Input: part model. Units: mm. Frame: model coordinates. Face numbers are marked on the shaded views. A direction names the side the tool comes from. Give positions to 0.01 mm unless a question says otherwise; leave off trailing zeros. Order: outer loops, then holes, each group sorted by start corner. A loop starts at its lowest first (then second) coordinate and runs counter-clockwise, first axis right, second up. Notation, with made-up numbers: M 17,-25.75 L 35,-25.75 A19 cw 35,-13.75 Z; hole C -28,62 d11. An arc over 180 degrees is marked long. Use a Markdown table: item, result.
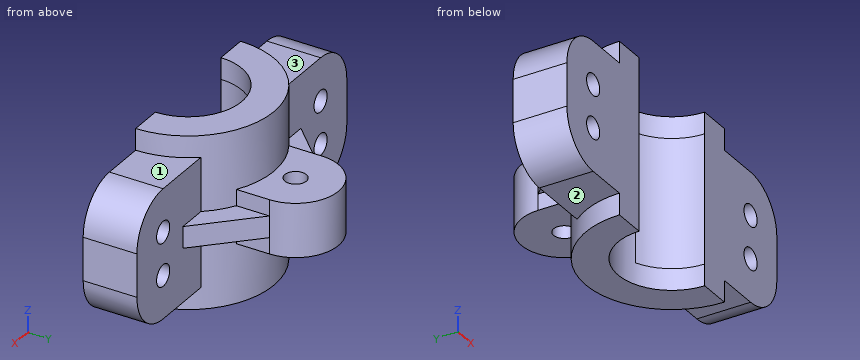
from build123d import *

# Parameters (mm, degrees)
BOSS_EXTRUDE1_DEPTH        = 40
SKETCH2_W                  = 70
SKETCH2_H                  = 60
BOSS_EXTRUDE2_DEPTH        = 25
FILLET1_R                  = 20
F_10_0_10_DIAMETER_HOLE1_D = 10
FILLET1_OF_MIRROR1_R       = 20
DELETEFACE1_START          = -30
DELETEFACE1_DEPTH          = 60
SKETCH5_R                  = 5
BOSS_EXTRUDE3_DEPTH        = 12.5015
RIB1_REACH                 = 115.578
SKETCH6_WALL_W             = 264.511672892
SKETCH6_WALL_H             = 10


# Read off the part's stored shape, not the designer's step: DeleteFace1
with BuildPart() as part:
    # Sketch1 → Boss-Extrude1 (new, symmetric)
    with BuildSketch(Plane.XY):
        with BuildLine():
            Line((-40, 0), (-25, 0))
            ThreePointArc((-25, 0), (0, 25), (25, 0))
            Line((25, 0), (40, 0))
            ThreePointArc((40, 0), (0, 40), (-40, 0))
        make_face()
    extrude(amount=BOSS_EXTRUDE1_DEPTH, both=True)

    # Sketch2 → Boss-Extrude2 (add)
    with BuildSketch(Plane.XZ):
        with Locations((-45, 0)):
            Rectangle(SKETCH2_W, SKETCH2_H)
    boss_extrude2 = extrude(amount=-BOSS_EXTRUDE2_DEPTH)

    # Fillet1
    fillet1_edges = [part.edges().sort_by_distance(p)[0] for p in [
        (-80, 12.5, 30),
        (-80, 12.5, -30),
    ]]
    fillet(fillet1_edges, radius=FILLET1_R)

    # Ø10.0 (10) Diameter Hole1 (through all)
    with Locations(Plane(origin=(0, 25, 0), x_dir=(1, 0, 0), z_dir=(0, 1, 0))):
        with Locations((-60, -10), (-60, 10)):
            f_10_0_10_diameter_hole1 = Hole(F_10_0_10_DIAMETER_HOLE1_D / 2)

    # Mirror1: Boss-Extrude2, Ø10.0 (10) Diameter Hole1 across plane
    add(boss_extrude2.mirror(Plane(origin=(0, 0, 0), x_dir=(0, 0, 1), z_dir=(1, 0, 0))))
    add(f_10_0_10_diameter_hole1.mirror(Plane(origin=(0, 0, 0), x_dir=(0, 0, 1), z_dir=(1, 0, 0))), mode=Mode.SUBTRACT)

    # Fillet1 of Mirror1
    fillet1_of_mirror1_edges = [part.edges().sort_by_distance(p)[0] for p in [
        (80, 12.5, 30),
        (80, 12.5, -30),
    ]]
    fillet(fillet1_of_mirror1_edges, radius=FILLET1_OF_MIRROR1_R)

    # DeleteFace1 outline → DeleteFace1 (cut)
    with BuildSketch(Plane.XY.offset(DELETEFACE1_START)):
        with BuildLine():
            ThreePointArc((25, 0), (20.916500663, 13.693063938), (10, 22.912878475))
            Line((10, 22.912878475), (10, 0))
            Line((10, 0), (25, 0))
        make_face()
        with BuildLine():
            ThreePointArc((-10, 22.912878475), (-20.916500663, 13.693063938), (-25, 0))
            Line((-25, 0), (-10, 0))
            Line((-10, 0), (-10, 22.912878475))
        make_face()
    extrude(amount=DELETEFACE1_DEPTH, mode=Mode.SUBTRACT)

    # Sketch5 → Boss-Extrude3 (add, symmetric)
    with BuildSketch(Plane.XY):
        with BuildLine():
            Line((-20, 50), (-20, 34.641016151))
            ThreePointArc((-20, 34.641016151), (0, 40), (20, 34.641016151))
            Line((20, 34.641016151), (20, 50))
            ThreePointArc((20, 50), (0, 70), (-20, 50))
        make_face()
        with Locations((0, 50)):
            Circle(SKETCH5_R, mode=Mode.SUBTRACT)
    extrude(amount=BOSS_EXTRUDE3_DEPTH, both=True)

    # Sketch6 wall → Rib1 (add, up to next)
    with BuildSketch(Plane(origin=(-32.5, 37.5, 0), x_dir=(0.707106781187, 0.707106781187, 0), z_dir=(-0.707106781187, 0.707106781187, 0)), mode=Mode.PRIVATE) as rib1_sk1:
        Rectangle(SKETCH6_WALL_W, SKETCH6_WALL_H)
    rib1_tool1 = extrude(rib1_sk1.sketch, amount=-RIB1_REACH, mode=Mode.PRIVATE) - part.part
    rib1 = rib1_tool1.solids().sort_by_distance((-32.5, 37.5, 0))[0]
    add(rib1)

    # Mirror2: Rib1 across plane
    add(rib1.mirror(Plane(origin=(0, 0, 0), x_dir=(0, 0, 1), z_dir=(1, 0, 0))))


solid = part.part
1) Cut plane D-D on y = 47. Return loops of the section in (x, z).
Response values:
| item | result |
|---|---|
| outline | M -23,-5 L -20,-5 L -20,-12.5 L -4,-12.5 L -4,12.5 L -20,12.5 L -20,5 L -23,5 Z; M 4,-12.5 L 20,-12.5 L 20,-5 L 23,-5 L 23,5 L 20,5 L 20,12.5 L 4,12.5 Z |
2) Material intervals for line 1 (Z direction, x = -60, y = 7); line 2 (X direction, y = 14.5, z = 7); line 3 (Y direction, x = -50.5, z = -13), sorted ascending. Write a range as from..to.
Response values:
| item | result |
|---|---|
| line 1 | z = -30..-15, -5..5, 15..30 |
| line 2 | x = -80..-64, -56..-20.37, 20.37..56, 64..80 |
| line 3 | y = 0..25 |
3) Cut plane B-B on x = 0. Return loops of the section in (y, z), and give its area (3 significant figures).
Response values:
| item | result |
|---|---|
| outline | M 25,-40 L 40,-40 L 40,-12.5 L 45,-12.5 L 45,12.5 L 40,12.5 L 40,40 L 25,40 Z; M 55,-12.5 L 70,-12.5 L 70,12.5 L 55,12.5 Z |
| area | 1,700 mm² |
4) First-contact query: pin 1 Ø2 at (y, z) = (39, 2.5) entering from -X; pin 2 Ø8.5 at (y, z) = (45, -9.5) entering from +X; pin 3 Ø2.5 at (y, z) = (42.5, -9.5) entering from -X. Flat tips, straight axial feed; report the tip coordinate or a pass-through.
Response values:
| item | result |
|---|---|
| pin 1 | stops at x = -32 |
| pin 2 | stops at x = 20 |
| pin 3 | stops at x = -20 |
5) Cut plane A-A on y = 20.5. Return loops of the section in (x, z), and give its area (3 significant figures).
Response values:
| item | result |
|---|---|
| outline | M -80,-10 A20 ccw -60,-30 L -34.35,-30 L -34.35,-40 L -14.31,-40 L -14.31,40 L -34.35,40 L -34.35,30 L -60,30 A20 ccw -80,10 Z; M 14.31,-40 L 34.35,-40 L 34.35,-30 L 60,-30 A20 ccw 80,-10 L 80,10 A20 ccw 60,30 L 34.35,30 L 34.35,40 L 14.31,40 Z; hole C -60,-10 d10; hole C -60,10 d10; hole C 60,-10 d10; hole C 60,10 d10 |
| area | 8,030 mm² |
6) Cut plane C-C on z = 2. Return loops of the section in (x, y).
Response values:
| item | result |
|---|---|
| outline | M -80,0 L -25,0 A25 cw 25,0 L 80,0 L 80,25 L 45,25 L 20,50 A20 ccw -20,50 L -45,25 L -80,25 Z; hole C 0,50 d10 |
7) Reachability of the marked faces 1, 2 and 3 from +Z, -Z, +X, -X, +Y, -Y: full face, straight path, thin tool, end or side. Return the list, or none.
Response values:
| item | result |
|---|---|
| face 1 | +Z, +X, +Y |
| face 2 | -Z, -X, +Y |
| face 3 | +Z, -X, +Y |
